The figure shows three views and two pictorial views of one solid part (mm, origin at its lowest corner). Answer the questions. A direction names the side the tool comes from. Coordinates: 2 decimals unless noted, no trailing zeros. Order: outer loops, then holes, each group sorted by start corner. A loop starts at its lowest first (then second) coordinate and runs counter-clockwise, first axis right, second up. Notation, with made-up numbers: (14.5, -16) -> (64.5, -16) arc R22 cw to (64.5, 22) -> close; hole circle Ø1 at (-22.75, 24). An arc over 180 degrees is marked (long way). Return JSON: item names as keys, results as strings.
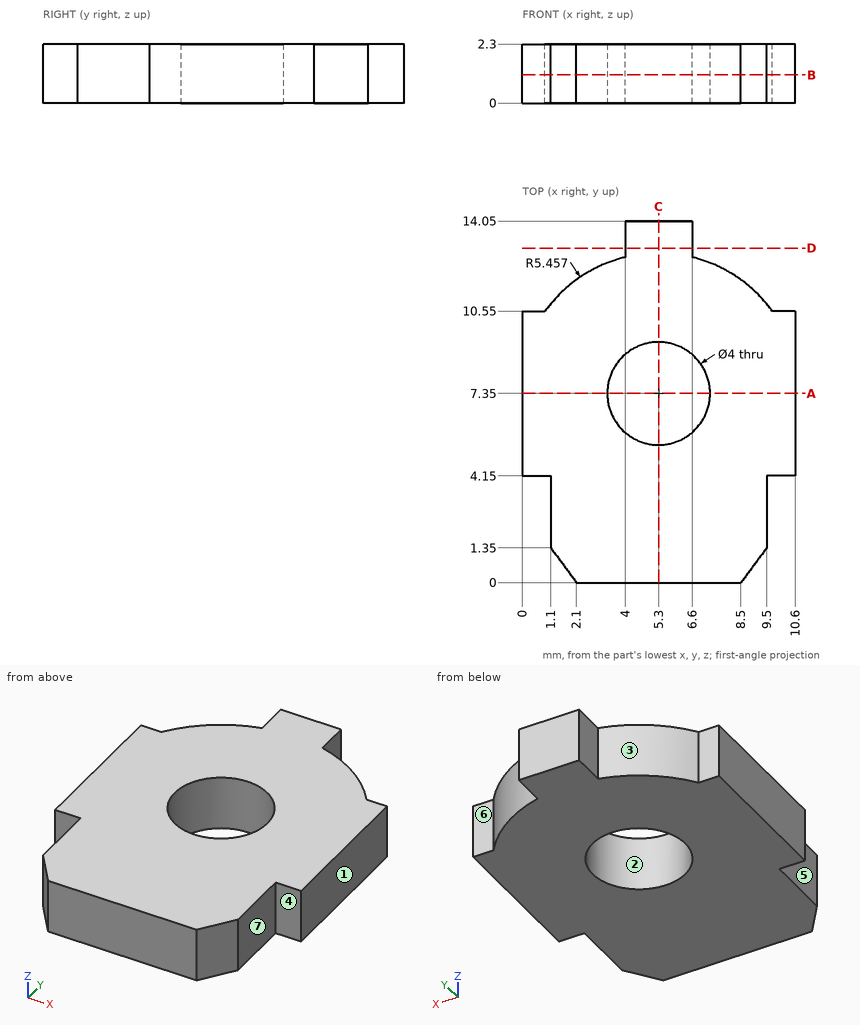
Item 1: Which of the six approach directions +Z, -Z, +X, -X, +Y, -Y give full straight-line access (tool end or side, diameter ignored) to the marked faces 5, 6 and 7?
Answer list:
{"face 5": "+Z, -Z, -X, -Y", "face 6": "+Z, -Z, +X, +Y", "face 7": "+Z, -Z, +X, -Y"}
Item 2: Flat-ended cylindrical pins translate along their axes: pin 1 (2.5 mm diameter, centred on x = 5.3, y = 7.35, fed in from +Z); pin 2 (0.9 mm diameter, centred on x = 0.5, z = 1, fed in from -Y); pin 3 (0.7 mm diameter, centred on x = 0.5, z = 1.5, fed in from +Y); pin 4 (1.1 mm diameter, centred on y = 13.5, z = 1, fed in from +X). Find the tip coordinate at first contact, or state that the pin passes through.
Answer list:
{"pin 1": "through", "pin 2": "y = 4.15", "pin 3": "y = 10.55", "pin 4": "x = 6.6"}
Item 3: The part is cut by section C-C on x = 5.3. Determine the outline of the cut face in (y, z).
Answer list:
{"outline": "(0, 0) -> (5.35, 0) -> (5.35, 2.3) -> (0, 2.3) -> close; (9.35, 0) -> (14.05, 0) -> (14.05, 2.3) -> (9.35, 2.3) -> close"}
Item 4: Determine the mould class of the marked faces 1, 2, 3 and 4 for opening direction X: pulls with the +X half, pulls with the -X half, needs draft (parallel to the pull), parting line crosses it, or undercut.
Answer list:
{"face 1": "pulls with the +X half", "face 2": "undercut", "face 3": "pulls with the -X half", "face 4": "needs draft"}
Item 5: The part is cut by section A-A on y = 7.35. Determine the outline of the cut face in (x, z).
Answer list:
{"outline": "(0, 0) -> (3.3, 0) -> (3.3, 2.3) -> (0, 2.3) -> close; (7.3, 0) -> (10.6, 0) -> (10.6, 2.3) -> (7.3, 2.3) -> close"}
Item 6: The part is cut by section B-B on z = 1.1. Determine the outline of the cut face in (x, y), plus the area to 3 significant figures.
Answer list:
{"outline": "(0, 4.15) -> (1.1, 4.15) -> (1.1, 1.35) -> (2.1, 0) -> (8.5, 0) -> (9.5, 1.35) -> (9.5, 4.15) -> (10.6, 4.15) -> (10.6, 10.55) -> (9.72, 10.55) arc R5.46 ccw to (6.6, 12.65) -> (6.6, 14.05) -> (4, 14.05) -> (4, 12.65) arc R5.46 ccw to (0.88, 10.55) -> (0, 10.55) -> close; hole circle Ø4 at (5.3, 7.35)", "area": "106 mm2"}
Item 7: The part is cut by section D-D on y = 13. Determine the outline of the cut face in (x, z).
Answer list:
{"outline": "(4, 0) -> (6.6, 0) -> (6.6, 2.3) -> (4, 2.3) -> close"}
Item 8: Find the intervals of material crossed by probe 1 along Y at (x, z) = (5.3, 1.75); probe 2 along Y at (x, z) = (6, 1.65); probe 3 along X at (y, z) = (2, 1.6), in increasing order.
Answer list:
{"probe 1": "0 to 5.35, 9.35 to 14.05", "probe 2": "0 to 5.48, 9.22 to 14.05", "probe 3": "1.1 to 9.5"}
